Build history of the part. All positions in model axes, mm. Give positions to 0.01 mm unless a question says otherwise; leave off trailing zeros. Write each loop counter-clockwise with the first axis right and the second up, starting at its lowest first coordinate (ties: lowest second). Pieces come first, ordered by that corner, then holes. Notation, with made-up numbers: M 24.25,57 L 45.25,57 A29 ccw 45.25,83 Z; hole C 23,66.25 d11. An arc over 180 degrees is marked long. One line per item, written item: value. Start each with the question number.
from build123d import *

# Parameters (mm, degrees)
BOSS_EXTRUDE1_DEPTH               = 10
SKETCH16_W                        = 20
SKETCH16_H                        = 440
BOSS_EXTRUDE2_DEPTH               = 10
SKETCH2_R                         = 1.55
SKETCH2_W                         = 60
SKETCH2_H                         = 323.65
SKETCH2_W_2                       = 10.2
SKETCH2_H_2                       = 10.2
CUT_EXTRUDE1_DEPTH                = 582.463670404
FILLET1_R                         = 20
SKETCH10_W                        = 25
SKETCH10_H                        = 100
WIRINGSLOT_DEPTH                  = 582.463670404
SKETCH6_R                         = 1.55
MOUNTINGHOLES_RAMPS_DEPTH         = 582.463670404
SKETCH5_R                         = 1.55
MOUNTINGHOLES_MELZI_DEPTH         = 582.463670404
SKETCH13_R                        = 1.55
MOUNTINGHOLES_SMOOTHIEBOARD_DEPTH = 582.463670404
SKETCH21_R                        = 1.55
PI_2_DEPTH                        = 582.463670404
CUT_EXTRUDE3_DEPTH                = 582.463670404
CUT_EXTRUDE4_DEPTH                = 582.463670404


with BuildPart() as part:
    # Sketch1 → Boss-Extrude1 (new body)
    with BuildSketch(Plane(origin=(0, 0, 0), x_dir=(1, 0, 0), z_dir=(0, 1, 0))):
        Polygon((0, 0), (-235, 0), (-235, -215), (-380, -352), (-380, -410), (-345, -440), (-293, -440), (-277, -405), (-212, -405), (-185.925501433, -440), (0, -440), align=None)
    extrude(amount=BOSS_EXTRUDE1_DEPTH)

    # Sketch16 → Boss-Extrude2 (add, through all)
    with BuildSketch(Plane(origin=(0, 10, 0), x_dir=(1, 0, 0), z_dir=(0, 1, 0))):
        with Locations((10, -220)):
            Rectangle(SKETCH16_W, SKETCH16_H)
    extrude(amount=-BOSS_EXTRUDE2_DEPTH)

    # Sketch2 → Cut-Extrude1 (cut, through all)
    with BuildSketch(Plane(origin=(0, 10, 0), x_dir=(1, 0, 0), z_dir=(0, 1, 0))):
        with Locations(Location((-16, -413, 0), (0, 0, 270))):
            Circle(SKETCH2_R)
        with Locations(Location((-16, -389, 0), (0, 0, 270))):
            Circle(SKETCH2_R)
        with Locations(Location((-355.55, -413, 0), (0, 0, 270))):
            Circle(SKETCH2_R)
        with Locations(Location((-355.55, -389, 0), (0, 0, 270))):
            Circle(SKETCH2_R)
        with Locations(Location((-174.5, -19.35, 0), (0, 0, 270))):
            Circle(SKETCH2_R)
        with Locations(Location((-134.5, -19.35, 0), (0, 0, 90))):
            Circle(SKETCH2_R)
        with Locations(Location((-124.5, -387.1, 0), (0, 0, 270))):
            Circle(SKETCH2_R)
        with Locations(Location((-184.5, -387.1, 0), (0, 0, 90))):
            Circle(SKETCH2_R)
        Polygon((-345, -348.509746257), (-235, -244.578711775), (-210.5, -244.578711775), (-210.5, -377), (-345, -377), align=None)
        with Locations((-154.5, -213.175)):
            Rectangle(SKETCH2_W, SKETCH2_H)
        with Locations((-16, -425)):
            Rectangle(SKETCH2_W_2, SKETCH2_H_2)
        with Locations((-16, -401)):
            Rectangle(SKETCH2_W_2, SKETCH2_H_2)
        with Locations((-355.55, -401)):
            Rectangle(SKETCH2_W_2, SKETCH2_H_2)
        with Locations((-174.5, -33.35)):
            Rectangle(SKETCH2_W_2, SKETCH2_H_2)
        with Locations((-134.5, -33.35)):
            Rectangle(SKETCH2_W_2, SKETCH2_H_2)
        with Locations((-174.5, -387.1)):
            Rectangle(SKETCH2_W_2, SKETCH2_H_2)
        with Locations((-134.5, -387.1)):
            Rectangle(SKETCH2_W_2, SKETCH2_H_2)
        with Locations((-184.5, -411.1)):
            Rectangle(SKETCH2_W_2, SKETCH2_H_2)
        with Locations((-124.5, -411.1)):
            Rectangle(SKETCH2_W_2, SKETCH2_H_2)
    extrude(amount=-CUT_EXTRUDE1_DEPTH, mode=Mode.SUBTRACT)

    # Fillet1
    fillet1_edges = [part.edges().sort_by_distance(p)[0] for p in [
        (-235, 5, 0),
        (20, 5, 0),
    ]]
    fillet(fillet1_edges, radius=FILLET1_R)

    # Sketch10 → WiringSlot (cut, through all)
    with BuildSketch(Plane(origin=(0, 10, 0), x_dir=(1, 0, 0), z_dir=(0, 1, 0))):
        with Locations((-52.25, -228.175)):
            Rectangle(SKETCH10_W, SKETCH10_H)
    extrude(amount=-WIRINGSLOT_DEPTH, mode=Mode.SUBTRACT)

    # Sketch6 → MountingHoles-RAMPS (cut, through all)
    with BuildSketch(Plane(origin=(0, 10, 0), x_dir=(1, 0, 0), z_dir=(0, 1, 0))):
        with Locations(Location((-76.35, -274.475, 0), (0, 0, 90))):
            Circle(SKETCH6_R)
        with Locations(Location((-76.35, -199.575, 0), (0, 0, 90))):
            Circle(SKETCH6_R)
        with BuildLine():
            Line((-26.6, -192.575), (-26.6, -199.575))
            ThreePointArc((-26.6, -199.575), (-28.15, -201.125), (-29.7, -199.575))
            Line((-29.7, -199.575), (-29.7, -192.575))
            ThreePointArc((-29.7, -192.575), (-28.15, -191.025), (-26.6, -192.575))
        make_face()
        with BuildLine():
            Line((-29.7, -282.075), (-29.7, -275.075))
            ThreePointArc((-29.7, -275.075), (-28.15, -273.525), (-26.6, -275.075))
            Line((-26.6, -275.075), (-26.6, -282.075))
            ThreePointArc((-26.6, -282.075), (-28.15, -283.625), (-29.7, -282.075))
        make_face()
    mountingholes_ramps = extrude(amount=-MOUNTINGHOLES_RAMPS_DEPTH, mode=Mode.SUBTRACT)

    # Mirror1: MountingHoles-RAMPS across plane
    add(mountingholes_ramps.mirror(Plane(origin=(-52.25, 0, 0), x_dir=(0, 0, 1), z_dir=(1, 0, 0))), mode=Mode.SUBTRACT)

    # Sketch5 → MountingHoles-Melzi (cut, through all)
    with BuildSketch(Plane(origin=(0, 10, 0), x_dir=(1, 0, 0), z_dir=(0, 1, 0))):
        with Locations(Location((-73.25, -127.675, 0), (0, 0, 270))):
            Circle(SKETCH5_R)
        with Locations(Location((-31.25, -127.675, 0), (0, 0, 90))):
            Circle(SKETCH5_R)
        with Locations(Location((-31.25, -328.675, 0), (0, 0, 270))):
            Circle(SKETCH5_R)
        with Locations(Location((-73.25, -328.675, 0), (0, 0, 90))):
            Circle(SKETCH5_R)
    extrude(amount=-MOUNTINGHOLES_MELZI_DEPTH, mode=Mode.SUBTRACT)

    # Sketch13 → Mountingholes-Smoothieboard (cut, through all)
    with BuildSketch(Plane(origin=(0, 0, 0), x_dir=(-1, 0, 0), z_dir=(0, -1, 0))):
        with Locations(Location((101.46, -163.66, 0), (0, 0, 90))):
            Circle(SKETCH13_R)
        with Locations(Location((101.46, -262.69, 0), (0, 0, 270))):
            Circle(SKETCH13_R)
        with Locations(Location((8.62, -170.14, 0), (0, 0, 90))):
            Circle(SKETCH13_R)
        with Locations(Location((3.56, -262.69, 0), (0, 0, 90))):
            Circle(SKETCH13_R)
    mountingholes_smoothieboard = extrude(amount=-MOUNTINGHOLES_SMOOTHIEBOARD_DEPTH, mode=Mode.SUBTRACT)

    # Flipped: Mountingholes-Smoothieboard across plane
    add(mountingholes_smoothieboard.mirror(Plane(origin=(-52.25, 0, 0), x_dir=(0, 0, 1), z_dir=(1, 0, 0))), mode=Mode.SUBTRACT)

    # Sketch21 → Pi 2 (cut, through all)
    with BuildSketch(Plane(origin=(0, 10, 0), x_dir=(1, 0, 0), z_dir=(0, 1, 0))):
        with Locations(Location((-27.75, -33.675, 0), (0, 0, 270))):
            Circle(SKETCH21_R)
        with Locations(Location((-76.75, -33.675, 0), (0, 0, 90))):
            Circle(SKETCH21_R)
        with Locations(Location((-76.75, -91.675, 0), (0, 0, 270))):
            Circle(SKETCH21_R)
        with Locations(Location((-27.75, -91.675, 0), (0, 0, 90))):
            Circle(SKETCH21_R)
    extrude(amount=-PI_2_DEPTH, mode=Mode.SUBTRACT)

    # Sketch17 → Cut-Extrude3 (cut, through all)
    with BuildSketch(Plane(origin=(0, 10, 0), x_dir=(1, 0, 0), z_dir=(0, 1, 0))):
        with BuildLine():
            Line((20, -14.5), (5, -14.5))
            ThreePointArc((5, -14.5), (0.5, -10), (5, -5.5))
            Line((5, -5.5), (20, -5.5))
            ThreePointArc((20, -5.5), (24.5, -10), (20, -14.5))
        make_face()
    extrude(amount=-CUT_EXTRUDE3_DEPTH, mode=Mode.SUBTRACT)

    # Sketch18 → Cut-Extrude4 (cut, through all)
    with BuildSketch(Plane(origin=(0, 10, 0), x_dir=(1, 0, 0), z_dir=(0, 1, 0))):
        with BuildLine():
            Line((9.5, -10), (9.5, -25))
            ThreePointArc((9.5, -25), (5, -29.5), (0.5, -25))
            Line((0.5, -25), (0.5, -10))
            ThreePointArc((0.5, -10), (5, -5.5), (9.5, -10))
        make_face()
    extrude(amount=-CUT_EXTRUDE4_DEPTH, mode=Mode.SUBTRACT)


solid = part.part
1) Band-saw the part on A-A (z = 368). List the corners of the cut face in (x, y), then the cut area to 4 significant figures.
2) Band-saw the part on D-D (y = 6.5). Count the separate pieces of the cut face and the enclosed holes in it, then the cut area to 3 significant figures.
3) Drop flat-ended pins along their axis: P1, Ø3, axis at y = 5.5, z = 427.5, coming from the -X side; P2, Ø5.5, axis at y = 3.5, z = 195.5, coming from the -X side. Give the stop position or say it passes through.
4) Band-saw the part on B-B (x = -48). List the corners of the cut face in (y, z) (3 decimals).
5) Probe line 1 along Z through (x, y) = (-176.5, 3); line 2 along X through (y, z) = (1.25, 179); line 3 along Z through (x, y) = (-76.75, 2.25) (1 decimal). List the from-to ranges inside material, lowest first. Write a range as from..to.
6) Mould opens along Z. For faces 1 (the face through (-306.485, 4.93, 282.541)), 2 (the face through (-362.745, 4.93, 424.79)), 3 (the face through (14, 5, 14.5)) say: released by +Z, released by -Z, zero draft, split by the parting line, or undercut.
7) Band-saw the part on C-C (z = 292.5). List the corners of the cut face in (x, y).
Model answer:
1. outline: M -380,0 L -345,0 L -345,10 L -380,10 Z; M -210.5,0 L -184.5,0 L -184.5,10 L -210.5,10 Z; M -124.5,0 L 20,0 L 20,10 L -124.5,10 Z
1. area: 2,055 mm²
2. separate pieces: 1
2. enclosed holes: 38
2. area: 95,700 mm²
3. P1: stops at x = -361.33
3. P2: stops at x = -235
4. outline: M 0,0 L 10,0 L 10,178.175 L 0,178.175 Z; M 0,278.175 L 10,278.175 L 10,440 L 0,440 Z
5. line 1: z = 0..28.25, 38.45..51.35, 375..382, 392.2..440
5. line 2: x = -235..-184.5, -124.5..-64.75, -39.75..20
5. line 3: z = 0..32.1, 35.2..90.1, 93.2..191.1, 201.1..273, 283.6..440
6. face 1: released by -Z
6. face 2: released by +Z
6. face 3: undercut
7. outline: M -317.03,0 L -285.72,0 L -285.72,10 L -317.03,10 Z; M -210.5,0 L -184.5,0 L -184.5,10 L -210.5,10 Z; M -124.5,0 L 20,0 L 20,10 L -124.5,10 Z
